Design review of the part built by this model. Coordinates are the model's own, in mm. Give positions to 0.01 mm unless a question says otherwise; leave off trailing zeros. Order: outer loops, then holes, each group sorted by start corner. A loop starts at its lowest first (then second) coordinate and runs counter-clockwise, first axis right, second up. Notation, with made-up numbers: (3, 26) -> (16, 26) arc R13 ccw to (16, 40) -> close; hole circle Ø8 at (82.25, -9.75). An arc over 180 degrees is marked (long way). One line per item, written item: value.
Autodesk Inventor part; units mm, degrees
ref_plane "YZ Plane" through (0, 0, 0) normal (1, 0, 0) x (0, 1, 0)
ref_plane "XZ Plane" through (0, 0, 0) normal (0, 1, 0) x (-1, 0, 0)
ref_plane "XY Plane" through (0, 0, 0) normal (0, 0, 1) x (1, 0, 0)
sketch "Sketch_1" plane through (0, 0, 0) normal (1, 0, 0) x (0, 1, 0)
  line L0 (0, 40) -> (0, 0)
  line L1 (0, 0) -> (40, 0)
  arc A0 (40, 0) -> (34, 6) centre (34, 0) ccw
  line L2 (34, 6) -> (12, 6)
  arc A1 (6, 12) -> (12, 6) centre (12, 12) ccw
  line L3 (6, 12) -> (6, 34)
  arc A2 (6, 34) -> (0, 40) centre (0, 34) ccw
extrude "Extrusion1" add sketch "Sketch_1" along normal mid plane 36
sketch "Sketch2" plane through (18, 40, 0) normal (0, 0, -1) x (-1, 0, 0)
  point P0 (18, -20)
hole "Hole1" at (0, 20, 0) direction (0, 0, 1) diameter 8.3 depth 6
sketch "Sketch3" plane through (-18, 0, 0) normal (0, -1, 0) x (1, 0, 0)
  point P0 (18, 20)
hole "Hole2" at (0, 0, 20) direction (0, 1, 0) diameter 8.3 depth 6
properties part number "40-4302 Aluminum"
Item 1: Add section D-D on x = 9.5. Give the boundary of the cut face in (y, z).
Returned:
outline: (0, 0) -> (40, 0) arc R6 ccw to (34, 6) -> (12, 6) arc R6 cw to (6, 12) -> (6, 34) arc R6 ccw to (0, 40) -> close
Item 2: Draft analysis for pull direction Y (two halves, no side actions). For faces 1 (the flat face through (0, 6, 25)), 2 (the flat face through (0, 26, 6)), 3 (the cylindrical face through (-0.182, 15.854, 3.042)), 4 (the flat face through (-4.3, 0, 20.3)), state which applies: pulls with the +Y half, pulls with the -Y half, needs draft (parallel to the pull), parting line crosses it, or undercut.
Returned:
face 1: pulls with the +Y half
face 2: needs draft
face 3: undercut
face 4: pulls with the -Y half
Item 3: Clearance check with flat-ended pins moving along their axes: P1, Ø1.5, axis at x = -12, y = 16, coming from the +Z side; P2, Ø8, axis at x = 10, y = 31, coming from the -Z side; P3, Ø1, axis at x = 6.5, z = 36, coming from the +Y side; P4, Ø17.5, axis at x = 7, z = 26.5, coming from the +Y side. State where each tip first meets the part, or that it passes through.
Returned:
P1: z = 6
P2: z = 0
P3: y = 5.81
P4: y = 6
Item 4: Add section C-C on x = 0. Give the boundary of the cut face in (y, z).
Returned:
outline: (0, 0) -> (15.85, 0) -> (15.85, 6) -> (12, 6) arc R6 cw to (6, 12) -> (6, 15.85) -> (0, 15.85) -> close; (0, 24.15) -> (6, 24.15) -> (6, 34) arc R6 ccw to (0, 40) -> close; (24.15, 0) -> (40, 0) arc R6 ccw to (34, 6) -> (24.15, 6) -> close
Item 5: Add section A-A on y = 20. Give the boundary of the cut face in (x, z).
Returned:
outline: (-18, 0) -> (-4.15, 0) -> (-4.15, 6) -> (-18, 6) -> close; (4.15, 0) -> (18, 0) -> (18, 6) -> (4.15, 6) -> close
Item 6: To check wall thickness, follow line 1 along X through (y, z) = (20, 3); line 2 along Z through (x, y) = (-6, 26). State the ranges of each line that lie inside material, in increasing order. Write a range as from..to.
Returned:
line 1: -18..-4.15, 4.15..18
line 2: 0..6
